Could you check a few things on this drawing? It's one solid part, dimensions in mm from its lowest x, y, z. Round coordinates to 2 decimals unless told otherwise and drop trailing zeros. Write each loop counter-clockwise with the first axis right and the second up, starting at its lowest first coordinate (ties: lowest second). Pieces come first, ordered by that corner, then holes. Notation, with made-up numbers: (82, 46) - (106, 46) arc R24 cw to (106, 73) - close; hole circle Ø3 at (25.5, -2). An arc over 180 degrees is marked (long way). One line per question, with ' | ' between items. Start each with the question number.
(1) If I drill on L1, parallel to Z at x = 8, y = 3.8; L2, parallel to Z at x = 36, y = 4.75 (1 decimal); L3, parallel to Y at x = 31.5, z = 4.95, over which ranges is the centre line in solid material (lowest first)?
(2) Imagine slicing it at A-A (z = 3). Write out the boundary of the cut face in (x, y) (1 decimal), plus the area to 3 significant figures.
(3) Imagine slicing it at C-C (x = 25.5). Write out the boundary of the cut face in (y, z).
(4) Will these pins go through, and if not, where does the flat tip stop? pin 1 (1 mm diameter, centred on x = 22, y = 2, fed in from -Z); pin 2 (1.5 mm diameter, centred on y = 2, z = 0.5, fed in from +X); pin 3 (1.5 mm diameter, centred on x = 25.5, y = 4.5, fed in from +Z) (1 decimal).
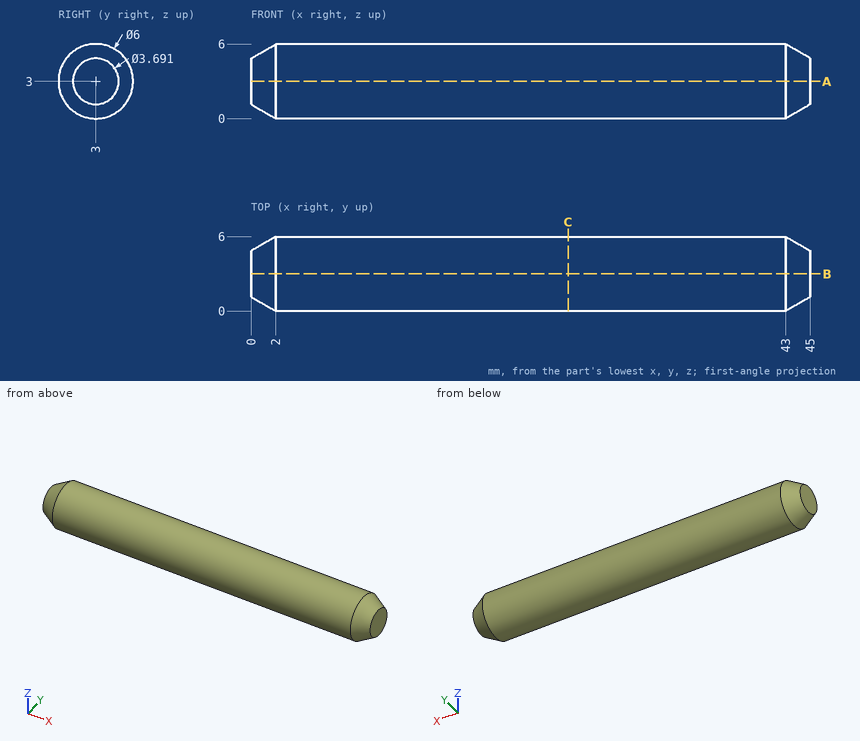
Check sheet entries:
1) L1: 0.11 to 5.89 | L2: 0.6 to 5.4 | L3: 0.72 to 5.28
2) outline: (0, 1.2) - (2, 0) - (43, 0) - (45, 1.2) - (45, 4.8) - (43, 6) - (2, 6) - (0, 4.8) - close | area: 265 mm^2
3) outline: circle Ø6 at (3, 3)
4) pin 1: z = 0.04 | pin 2: x = 44.83 | pin 3: z = 5.9
